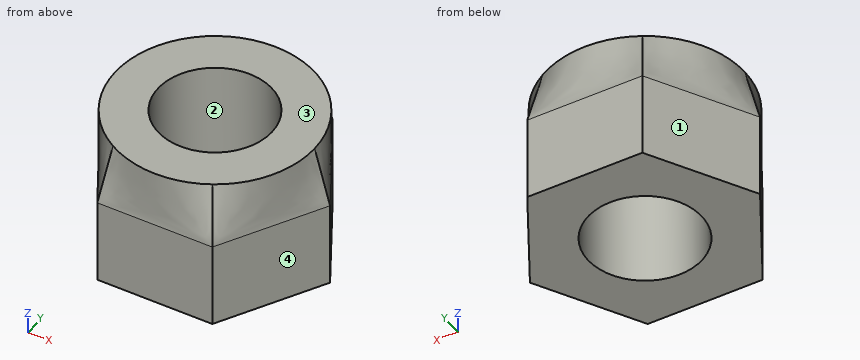
Autodesk Inventor part; units mm, degrees
ref_plane "Work Plane1" through (0, 0, 6.35) normal (0, 0, 1) x (1, 0, 0)
ref_plane "YZ Plane" through (0, 0, 0) normal (1, 0, 0) x (0, 1, 0)
ref_plane "XZ Plane" through (0, 0, 0) normal (0, 1, 0) x (-1, 0, 0)
sketch "Sketch1" plane through (0, 0, 0) normal (0, 0, 1) x (1, 0, 0)
  line L0 (2.5663, 4.445) -> (5.1326, 0)
  line L1 (5.1326, 0) -> (2.5663, -4.445)
  line L2 (2.5663, -4.445) -> (-2.5663, -4.445)
  line L3 (-2.5663, -4.445) -> (-5.1326, 0)
  line L4 (-5.1326, 0) -> (-2.5663, 4.445)
  line L5 (-2.5663, 4.445) -> (2.5663, 4.445)
  line L6 (0, 0) -> (0.7817, 0)
  dimension "d0" = 8.89
extrude "Extrusion1" add sketch "Sketch1" along normal blind 3.81
sketch "Sketch2" plane through (0, 0, 3.81) normal (0, 0, 1) x (1, 0, 0)
  line L0 (5.1326, 0) -> (2.5663, 4.445)
  line L1 (2.5663, 4.445) -> (-2.5663, 4.445)
  line L2 (-2.5663, 4.445) -> (-5.1326, 0)
  line L3 (-5.1326, 0) -> (-2.5663, -4.445)
  line L4 (-2.5663, -4.445) -> (2.5663, -4.445)
  line L5 (2.5663, -4.445) -> (5.1326, 0)
  point P0 (0, 0)
ref_plane "Work Plane1" through (0, 0, 6.35) normal (0, 0, 1) x (1, 0, 0)
sketch "Sketch3" plane through (0, 0, 6.35) normal (0, 0, 1) x (1, 0, 0)
  circle A0 centre (0, 0) radius 4.445
  dimension "d4" = 8.89
loft "Loft1" add profiles "Sketch2", "Sketch3"
sketch "Sketch4" plane through (0, 0, 6.35) normal (0, 0, 1) x (1, 0, 0)
  circle A0 centre (0, 0) radius 2.54
  dimension "d9" = 5.08
extrude "Extrusion2" cut sketch "Sketch4" against normal blind 25.4
properties part number "RobotArm Nut2"
Could you check a few things on this model? Use its own coordinates, in mm. Face numbers are marked on the shaded views. Coordinates: 2 decimals unless noted, no trailing zeros. Order: outer loops, then holes, each group sorted by start corner. A loop starts at its lowest first (then second) coordinate and runs counter-clockwise, first axis right, second up. Notation, with made-up numbers: (7.5, 32.5) -> (64.5, 32.5) arc R15 ccw to (64.5, 42.5) -> close; hole circle Ø7 at (57, 24.25). An arc over 180 degrees is marked (long way). One line per question, with ' | ' between items.
Q1. If I drill on L1, parallel to Y at x = 0, z = 4.5 (3 decimals); L2, parallel to Y at x = 1.25, z = 2.25 (3 decimals); L3, parallel to X at y = -1.5, z = 3.25, over which ranges is the centre line in solid material (lowest first)?
Return value:
L1: -4.445 to -2.54, 2.54 to 4.445 | L2: -4.445 to -2.211, 2.211 to 4.445 | L3: -4.27 to -2.05, 2.05 to 4.27
Q2. I'm going to push flat-ended pins straight in: P1, Ø1, axis at y = 3.5, z = 2, coming from the -X side; P2, Ø3, axis at y = 3, z = 3, coming from the +X side. Where does each tip first touch, or does it pass through?
Return value:
P1: x = -3.4 | P2: x = 4.27
Q3. Imagine slicing it at A-A on z = 3. Please give me the cut outline in (x, y) (3 decimals).
Return value:
outline: (-5.133, 0) -> (-2.566, -4.445) -> (2.566, -4.445) -> (5.133, 0) -> (2.566, 4.445) -> (-2.566, 4.445) -> close; hole circle Ø5.08 at (0, 0)
Q4. Thinking about a two-plate mould opening in X: for the marked faces 1, 2, 3 and 4, which applies, pulls with the +X half, pulls with the -X half, needs draft (parallel to the pull), parting line crosses it, or undercut?
Return value:
face 1: pulls with the -X half | face 2: undercut | face 3: needs draft | face 4: pulls with the +X half
